Model file for the job. Use its own axes, mm. Give positions to 0.01 mm unless a question says otherwise; leave off trailing zeros. Write each loop counter-clockwise with the first axis right and the second up, starting at its lowest first coordinate (ties: lowest second). Pieces come first, ordered by that corner, then holes. Notation, with made-up numbers: (26, 12) - (65, 12) arc R22 cw to (65, 45) - close; hole circle Ø7 at (18, 61). An arc over 180 degrees is marked (long way). One line per item, written item: value. Start each with the question number.
(1) Drop flat-ended pins along their axis: P1, Ø0.8, axis at y = 8.5, z = 38, coming from the +X side; P2, Ø0.8, axis at y = 8.5, z = -53, coming from the -X side; P3, Ø10, axis at x = -29.5, z = -35, coming from the -Y side; P4, Ø3, axis at x = 244.5, z = -25, coming from the +Y side. Give the stop position or say it passes through.
(2) Cut at A-A, the plane y = 15. List the corners of the cut face in (x, z).
(3) Probe L1, parallel to Y at x = -31, z = 37; L2, parallel to Z at x = -50, y = 18.5. List the from-to ranges inside material, lowest first.
(4) Cut at C-C, the plane x = -81. List the corners of the cut face in (y, z), and give its area (3 significant figures).
(5) Cut at B-B, the plane z = 96. List the corners of the cut face in (x, y).
from build123d import *

# Parameters (mm, degrees)
SKETCH_1_W          = 430.43
SKETCH_1_H          = 250
EXTRUDE_1_DEPTH     = 10
SKETCH_2_W          = 250
SKETCH_2_H          = 6
EXTRUDE_2_DEPTH     = 10
SKETCH_3_W          = 150
SKETCH_3_H          = 20
EXTRUDE_3_DEPTH     = 30
CHAMFER_2_SIZE      = 10
CHAMFER_3_SIZE      = 10
CUT_EXTRUDE_2_DEPTH = 30


with BuildPart() as part:
    # 草图1 → 凸台-拉伸1 (new body)
    with BuildSketch(Plane(origin=(0, 0, 0), x_dir=(1, 0, 0), z_dir=(0, 1, 0))):
        with Locations((22.318592593, -1.184950617)):
            Rectangle(SKETCH_1_W, SKETCH_1_H)
    extrude(amount=EXTRUDE_1_DEPTH)

    # 草图2 → 凸台-拉伸2 (add)
    with BuildSketch(Plane(origin=(237.533592593, 0, 0), x_dir=(0, 0, -1), z_dir=(1, 0, 0))):
        with Locations((-1.184950617, 4.5)):
            Rectangle(SKETCH_2_W, SKETCH_2_H)
    extrude_2 = extrude(amount=EXTRUDE_2_DEPTH)

    # 镜向1: 凸台-拉伸2 across plane
    add(extrude_2.mirror(Plane(origin=(22.318592593, 0, 0), x_dir=(0, 0, 1), z_dir=(1, 0, 0))))

    # 草图3 → 凸台-拉伸3 (add)
    with BuildSketch(Plane(origin=(0, 10, 0), x_dir=(1, 0, 0), z_dir=(0, 1, 0))):
        with Locations((22.318592593, -96.184950617)):
            Rectangle(SKETCH_3_W, SKETCH_3_H)
    extrude(amount=EXTRUDE_3_DEPTH)

    # 倒角2
    chamfer_2_edges = [part.edges().sort_by_distance(p)[0] for p in [
        (97.318592593, 40, 96.184950617),
    ]]
    chamfer(chamfer_2_edges, length=CHAMFER_2_SIZE)

    # 倒角3
    chamfer_3_edges = [part.edges().sort_by_distance(p)[0] for p in [
        (-52.681407407, 40, 96.184950617),
    ]]
    chamfer(chamfer_3_edges, length=CHAMFER_3_SIZE)

    # 草图5 → 切除-拉伸2 (cut)
    with BuildSketch(Plane(origin=(0, 0, 86.184950617), x_dir=(-1, 0, 0), z_dir=(0, 0, -1))):
        Polygon((-87.318592593, 20), (-87.318592593, 10), (42.681407407, 10), (42.681407407, 20), (42.681407407, 25.857864376), (38.539271784, 30), (-83.176456969, 30), (-87.318592593, 25.857864376), align=None)
    extrude(amount=-CUT_EXTRUDE_2_DEPTH, mode=Mode.SUBTRACT)


solid = part.part
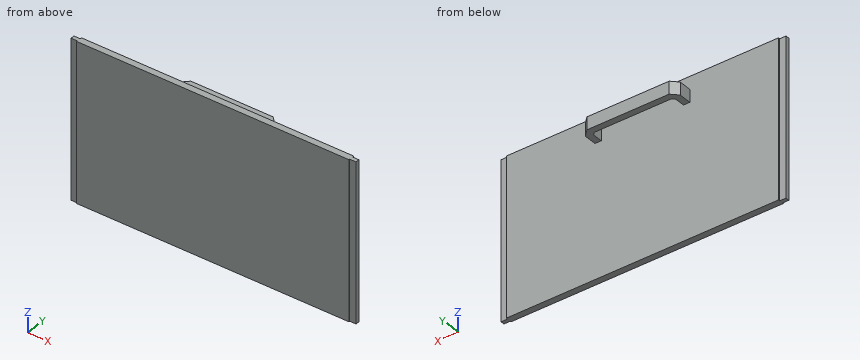
Answers follow:
1. P1: stops at x = 237.53
1. P2: stops at x = -192.9
1. P3: stops at y = 0
1. P4: stops at y = 7.5
2. outline: (-52.68, 86.18) - (-42.68, 86.18) - (-42.68, 106.18) - (-52.68, 106.18) - close; (87.32, 86.18) - (97.32, 86.18) - (97.32, 106.18) - (87.32, 106.18) - close
3. L1: y = 0 to 10
3. L2: z = 86.18 to 106.18
4. outline: (0, -123.82) - (10, -123.82) - (10, 126.18) - (0, 126.18) - close
4. area: 2,500 mm²
5. outline: (-202.9, 1.5) - (-192.9, 1.5) - (-192.9, 0) - (237.53, 0) - (237.53, 1.5) - (247.53, 1.5) - (247.53, 7.5) - (237.53, 7.5) - (237.53, 10) - (97.32, 10) - (97.32, 30) - (87.32, 40) - (-42.68, 40) - (-52.68, 30) - (-52.68, 10) - (-192.9, 10) - (-192.9, 7.5) - (-202.9, 7.5) - close; hole (-42.68, 10) - (87.32, 10) - (87.32, 25.86) - (83.18, 30) - (-38.54, 30) - (-42.68, 25.86) - close
